Autodesk Inventor part; units mm, degrees
ref_plane "Work Plane1" through (0, 0, 21.59) normal (0, 0, 1) x (1, 0, 0)
ref_plane "Work Plane2" through (-6.35, 0, 0) normal (-1, 0, 0) x (0, -1, 0)
ref_plane "YZ Plane" through (0, 0, 0) normal (1, 0, 0) x (0, 1, 0)
sketch "Sketch1" plane through (0, 0, 0) normal (0, 0, 1) x (1, 0, 0)
  circle A0 centre (0, 0) radius 6.35
  line L0 (8.382, -8.382) -> (-8.382, -8.382)
  line L1 (-8.382, -8.382) -> (-8.382, 8.382)
  line L2 (-8.382, 8.382) -> (8.382, 8.382)
  line L3 (8.382, 8.382) -> (8.382, -8.382)
  dimension "d10" = 12.7
  dimension "d11" = 2.032
  dimension "d26" = 16.764
  dimension "d28" = 0
  dimension "d29" = 8.382
  dimension "d37" = 2.032
  dimension "d38" = 2.032
  dimension "d39" = 2.032
extrude "Extrusion2" add sketch "Sketch1" along normal blind 25.4
sketch "Sketch2" plane through (-8.382, -8.382, 0) normal (-1, 0, 0) x (0, 0, 1)
  line L0 (25.4, 14.732) -> (25.4, 2.032)
  line L1 (0, 2.032) -> (0, 14.732)
  line L2 (0, 14.732) -> (25.4, 14.732)
  line L3 (0, 2.032) -> (25.4, 2.032)
  line L4 (0, 0) -> (0, 16.764)
  line L5 (0, 0) -> (25.4, 0)
  line L6 (25.4, 16.764) -> (25.4, 0)
  line L7 (0, 16.764) -> (25.4, 16.764)
  circle A0 centre (6.35, 15.748) radius 1.4224
  circle A1 centre (6.35, 1.016) radius 1.4224
  point P0 (0, 8.382)
  dimension "d17" = 2.032
  dimension "d18" = 2.8448
  dimension "d19" = 2.8448
  dimension "d20" = 1.016
  dimension "d21" = 1.016
  dimension "d22" = 6.35
  dimension "d23" = 6.35
extrude "Extrusion3" [suppressed]
sketch "Sketch3" plane through (0, 0, 0) normal (0, 0, -1) x (-1, 0, 0)
  circle A0 centre (0, 0) radius 3.3655
  circle A1 centre (0, 0) radius 6.35
  dimension "d30" = 6.731
extrude "Extrusion4" add sketch "Sketch3" against normal blind 2.54
ref_plane "Work Plane1" through (0, 0, 21.59) normal (0, 0, 1) x (1, 0, 0)
sketch "Sketch4" plane through (0, 0, 21.59) normal (0, 0, 1) x (1, 0, 0)
  circle A0 centre (0, 0) radius 6.35
  circle A1 centre (0, 0) radius 6.7056
  dimension "d34" = 0.3556
extrude "Extrusion5" cut sketch "Sketch4" along normal blind 1.016
sketch "Sketch5" plane through (-8.382, -8.382, 0) normal (-1, 0, 0) x (0, 0, 1)
  line L0 (0, 0) -> (0, 16.764)
  line L1 (0, 0) -> (25.4, 0)
  line L2 (25.4, 16.764) -> (25.4, 0)
  line L3 (0, 16.764) -> (25.4, 16.764)
  line L4 (25.4, 14.732) -> (25.4, 2.032)
  line L5 (21.59, 2.032) -> (21.59, 14.732)
  line L6 (2.54, 14.732) -> (2.54, 2.032)
  line L7 (0, 16.764) -> (25.4, 16.764)
  line L8 (6.35, 0) -> (12.7, 0)
  line L9 (12.7, 0) -> (12.7, 16.764)
  line L10 (12.7, 16.764) -> (6.35, 16.764)
  line L11 (6.35, 16.764) -> (6.35, 0)
  point P0 (0, 8.382)
  dimension "d40" = 6.35
  dimension "d41" = 6.35
ref_plane "Work Plane2" through (-6.35, 0, 0) normal (-1, 0, 0) x (0, -1, 0)
extrude "Extrusion6" cut sketch "Sketch5" against normal blind 1.27 contours L11 L3 L9 L1
sketch "Sketch7" plane through (0, 0, 0) normal (0, 0, -1) x (-1, 0, 0)
  line L0 (7.112, -8.382) -> (7.112, 8.382)
  line L1 (7.112, 8.382) -> (7.112, -8.382)
  point P0 (0, 0)
  dimension "d46" = 7.112
sketch "Sketch8" plane through (0, 0, 25.4) normal (0, 0, 1) x (1, 0, 0)
  circle A0 centre (0, 0) radius 6.35
  circle A1 centre (0, 0) radius 6.7056
  circle A2 centre (0, 0) radius 6.7056
  line L0 (8.382, -8.382) -> (-8.382, -8.382)
  line L1 (-8.382, 8.382) -> (8.382, 8.382)
  line L2 (8.382, 8.382) -> (8.382, -8.382)
  line L3 (5.334, 8.382) -> (8.382, 8.382)
  line L4 (8.382, 8.382) -> (8.382, -8.382)
  line L5 (8.382, -8.382) -> (5.334, -8.382)
  line L6 (5.334, -8.382) -> (5.334, 8.382)
  point P0 (5.207, -8.382)
  point P1 (5.207, -8.382)
  point P2 (-5.207, -8.382)
  dimension "d50" = 3.048
extrude "Extrusion8" cut sketch "Sketch8" against normal through all contours A0 L6 | A0 L6 A1 | L6 L1 L2 L0 A1 picked at (5.5198, -0.7897) picked at (6.4961, 0.8835)
fillet "Fillet3" radius 3.175 2 edges at (5.334, -8.382, 12.7) (5.334, 8.382, 12.7)
equation "\"d37\" = d11"
equation "\"d38\" = d11"
equation "\"d39\" = d11"
equation "\"d20\" = 0.5 * d17"
equation "\"d21\" = d20"
equation "\"d23\" = d22"
properties part number "linear bearing mount" material "Aluminum 6061"
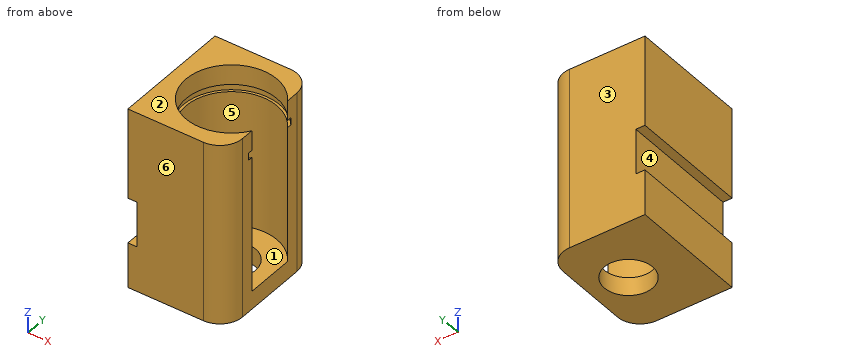
Source: CAD feature listing. Evaluate the final solid. Frame: model axes, mm. Face numbers are marked on the shaded views. A direction names the side the tool comes from. Give positions to 0.01 mm unless a question says otherwise; leave off trailing zeros. Order: outer loops, then holes, each group sorted by start corner. A loop starts at its lowest first (then second) coordinate and runs counter-clockwise, first axis right, second up.
(1) Section query B-B (y = 0). Return the cut outline in (x, z).
(2) Material intervals for line 1 along Y through (x, z) = (0, 0.65); line 2 along Y through (x, z) = (0, 8); line 3 along Z through (x, y) = (-0.5, 5.75), sorted ascending.
(3) Section query C-C (z = 21). Return the cut outline in (x, y) (3 decimals), plus the area to 3 significant figures.
(4) Pull-direction query (Y, two-part tool) for the marked faces 1, 2 and 3; classes: +Y half, -Y half, draft (parallel to the pull), parting line (faces both ways), or undercut.
(5) Contact query for a flat-ended pin moving along its axis: P1, Ø6, axis at x = -1.5, y = -2, coming from the +Z side. Output: stop coordinate, or through.
(6) Access query for the marked faces 4, 5 and 6. Directions: +Z, -Z, +X, -X, +Y, -Y. A direction counts if a zero-diameter tool reaches every point of the face in a straight line with its end or side. Return the directions, or none.
(7) Section query A-A (x = 0). Return the cut outline in (y, z).
(8) Section query D-D (x = -4). Return the cut outline in (y, z), plus the area to 3 significant figures.
Outcome:
1. outline: (-8.38, 0) - (-3.37, 0) - (-3.37, 2.54) - (-6.35, 2.54) - (-6.35, 21.59) - (-6.71, 21.59) - (-6.71, 22.61) - (-6.35, 22.61) - (-6.35, 25.4) - (-8.38, 25.4) - (-8.38, 12.7) - (-7.11, 12.7) - (-7.11, 6.35) - (-8.38, 6.35) - close; (3.37, 0) - (5.33, 0) - (5.33, 2.54) - (3.37, 2.54) - close
2. line 1: y = -8.38 to -3.37, 3.37 to 8.38
2. line 2: y = -8.38 to -6.35, 6.35 to 8.38
2. line 3: z = 0 to 2.54
3. outline: (-8.382, -8.382) - (2.159, -8.382) arc R3.175 ccw to (5.334, -5.207) - (5.334, -3.445) arc R6.35 cw (long way) to (5.334, 3.445) - (5.334, 5.207) arc R3.175 ccw to (2.159, 8.382) - (-8.382, 8.382) - close
3. area: 104 mm2
4. face 1: undercut
4. face 2: draft
4. face 3: +Y half
5. P1: stops at z = 2.54
6. face 4: -X, +Y, -Y
6. face 5: +Z
6. face 6: +Z, -Z, +X, -X, -Y
7. outline: (-8.38, 0) - (-3.37, 0) - (-3.37, 2.54) - (-6.35, 2.54) - (-6.35, 21.59) - (-6.71, 21.59) - (-6.71, 22.61) - (-6.35, 22.61) - (-6.35, 25.4) - (-8.38, 25.4) - close; (3.37, 0) - (8.38, 0) - (8.38, 25.4) - (6.35, 25.4) - (6.35, 22.61) - (6.71, 22.61) - (6.71, 21.59) - (6.35, 21.59) - (6.35, 2.54) - (3.37, 2.54) - close
8. outline: (-8.38, 0) - (8.38, 0) - (8.38, 25.4) - (4.93, 25.4) - (4.93, 22.61) - (5.38, 22.61) - (5.38, 21.59) - (4.93, 21.59) - (4.93, 2.54) - (-4.93, 2.54) - (-4.93, 21.59) - (-5.38, 21.59) - (-5.38, 22.61) - (-4.93, 22.61) - (-4.93, 25.4) - (-8.38, 25.4) - close
8. area: 199 mm2
